Part model, mm, in its own coordinate system. A direction names the side the tool comes from. Round coordinates to 2 decimals unless told otherwise and drop trailing zeros. Write each loop counter-clockwise with the first axis right and the second up, starting at its lowest first coordinate (ties: lowest second). Pieces come first, ordered by that corner, then holes.
```python
from build123d import *

# Parameters (mm, degrees)
SKETCH1_W                                        = 90
SKETCH1_H                                        = 60
BOSS_EXTRUDE1_DEPTH                              = 12.7
CSK_FOR_1_4_FLAT_HEAD_MACHINE_SCREW1_D           = 6.5278
CSK_FOR_1_4_FLAT_HEAD_MACHINE_SCREW1_CSINK_D     = 12.8778
CSK_FOR_1_4_FLAT_HEAD_MACHINE_SCREW1_CSINK_ANGLE = 82
FILLET1_R                                        = 2
CUT_EXTRUDE1_DEPTH                               = 109.909549627


with BuildPart() as part:
    # Sketch1 → Boss-Extrude1 (new body)
    with BuildSketch(Plane.XY):
        with Locations((45, -30)):
            Rectangle(SKETCH1_W, SKETCH1_H)
        Polygon((29.025, -3.367091904), (29.025, -16.267091904), (60.975, -16.267091904), (60.975, -3.367091904), (45, -3.367091904), align=None, mode=Mode.SUBTRACT)
    extrude(amount=BOSS_EXTRUDE1_DEPTH)

    # CSK for 1/4 Flat Head Machine Screw1 (through all)
    with Locations(Plane(origin=(0, 0, 0), x_dir=(-1, 0, 0), z_dir=(0, 0, -1))):
        with Locations((-82.49, -9.717091904), (-7.51, -9.717091904)):
            CounterSinkHole(CSK_FOR_1_4_FLAT_HEAD_MACHINE_SCREW1_D / 2, CSK_FOR_1_4_FLAT_HEAD_MACHINE_SCREW1_CSINK_D / 2, counter_sink_angle=CSK_FOR_1_4_FLAT_HEAD_MACHINE_SCREW1_CSINK_ANGLE)

    # Fillet1
    fillet1_edges = [part.edges().sort_by_distance(p)[0] for p in [
        (0, 0, 6.35),
        (90, 0, 6.35),
        (90, -60, 6.35),
        (0, -60, 6.35),
    ]]
    fillet(fillet1_edges, radius=FILLET1_R)

    # Sketch5 → Cut-Extrude1 (cut, through all)
    with BuildSketch(Plane(origin=(0, 0, 0), x_dir=(-1, 0, 0), z_dir=(0, 0, -1))):
        with BuildLine():
            Line((-10.785, -22.847364981), (-10.785, -52.847364981))
            ThreePointArc((-10.785, -52.847364981), (-7.485, -56.147364981), (-4.185, -52.847364981))
            Line((-4.185, -52.847364981), (-4.185, -22.847364981))
            ThreePointArc((-4.185, -22.847364981), (-7.485, -19.547364981), (-10.785, -22.847364981))
        make_face()
        with BuildLine():
            Line((-79.215, -52.847364981), (-79.215, -22.847364981))
            ThreePointArc((-79.215, -22.847364981), (-82.515, -19.547364981), (-85.815, -22.847364981))
            Line((-85.815, -22.847364981), (-85.815, -52.847364981))
            ThreePointArc((-85.815, -52.847364981), (-82.515, -56.147364981), (-79.215, -52.847364981))
        make_face()
    extrude(amount=-CUT_EXTRUDE1_DEPTH, mode=Mode.SUBTRACT)


solid = part.part
```
Q1. Drop flat-ended pins along their axis: pin 1 (4 mm diameter, centred on x = 82.49, y = -9.72, fed in from +Z); pin 2 (4 mm diameter, centred on x = 66.5, y = -9.5, fed in from -Z). Give the stop position or say it passes through.
Values follow:
pin 1: passes through
pin 2: stops at z = 0
Q2. Mould opens along X. For faces 3 (the cylindrical face through (0.57, -59.4, 6.44)), 4 (the cylindrical face through (10.525, -10.967, 8.24)), 5 (the flat face through (29.025, -10, 6)), 6 (the cylindrical face through (89.43, -59.4, 6.44)) say: +X half, -X half, draft (parallel to the pull), parting line (faces both ways), or undercut.
Values follow:
face 3: -X half
face 4: undercut
face 5: undercut
face 6: +X half
Q3. Wall check: L1, parallel to X at y = -40.5, z = 11.5 (3 decimals); L2, parallel to Y at x = 82.49, z = 10.25; L3, parallel to Y at x = 9, z = 3.5. Give the ranges that are in metal, low to high.
Values follow:
L1: x = 0 to 4.185, 10.785 to 79.215, 85.815 to 90
L2: y = -60 to -56.15, -19.55 to -12.98, -6.45 to 0
L3: y = -60 to -55.78, -19.92 to -12.77, -6.66 to 0
Q4. Cut at D-D on z = 8. Write the cut outline in (x, y) (3 decimals), plus the area to 3 significant figures.
Values follow:
outline: (0, -58) arc R2 ccw to (2, -60) - (88, -60) arc R2 ccw to (90, -58) - (90, -2) arc R2 ccw to (88, 0) - (2, 0) arc R2 ccw to (0, -2) - close; hole (4.185, -52.847) arc R3.3 ccw to (10.785, -52.847) - (10.785, -22.847) arc R3.3 ccw to (4.185, -22.847) - close; hole circle Ø6.528 at (7.51, -9.717); hole (29.025, -16.267) - (60.975, -16.267) - (60.975, -3.367) - (29.025, -3.367) - close; hole (79.215, -52.847) arc R3.3 ccw to (85.815, -52.847) - (85.815, -22.847) arc R3.3 ccw to (79.215, -22.847) - close; hole circle Ø6.528 at (82.49, -9.717)
area: 4,450 mm2
Q5. Cut at C-C on x = 7.51. Write the cut outline in (y, z).
Values follow:
outline: (-60, 0) - (-56.15, 0) - (-56.15, 12.7) - (-60, 12.7) - close; (-19.55, 0) - (-16.16, 0) - (-12.98, 3.65) - (-12.98, 12.7) - (-19.55, 12.7) - close; (-6.45, 3.65) - (-3.28, 0) - (0, 0) - (0, 12.7) - (-6.45, 12.7) - close
Q6. Cut at B-B on y = -46. Write the cut outline in (x, z) (3 decimals).
Values follow:
outline: (0, 0) - (4.185, 0) - (4.185, 12.7) - (0, 12.7) - close; (10.785, 0) - (79.215, 0) - (79.215, 12.7) - (10.785, 12.7) - close; (85.815, 0) - (90, 0) - (90, 12.7) - (85.815, 12.7) - close
Q7. Which spindle directions (+Z, -Z, +X, -X, +Y, -Y) get a long thin tool onto all of the face, cutting with end or side? Do faces 1 (the flat face through (10.785, -38, 6)), 2 (the cylindrical face through (0.57, -0.6, 6.44)). Say none if no direction does.
Values follow:
face 1: +Z, -Z
face 2: +Z, -Z, -X, +Y
Q8. Cut at A-A on x = 38.5. Write the cut outline in (y, z), plus the area to 3 significant figures.
Values follow:
outline: (-60, 0) - (-16.27, 0) - (-16.27, 12.7) - (-60, 12.7) - close; (-3.37, 0) - (0, 0) - (0, 12.7) - (-3.37, 12.7) - close
area: 598 mm2
